Read the model definition and answer for the solid it produces. Units are mm, in the model's axes. A direction names the side the tool comes from. Give positions to 0.01 mm unless a question says otherwise; leave off trailing zeros. Write each loop counter-clockwise with the first axis right and the second up, starting at its lowest first coordinate (ties: lowest second). Pieces come first, ordered by that corner, then holes. Notation, with made-up numbers: (-22.5, -35) -> (26.5, -35) arc R11 cw to (26.5, -21) -> close; hole circle Ø4 at (60.25, 66). An arc over 180 degrees is marked (long way). Use a Markdown table: item, result.
from build123d import *

# Parameters (mm, degrees)
SKETCH_1_R          = 1.7
EXTRUDE_1_DEPTH     = 10
SKETCH_2_R          = 1.7
EXTRUDE_2_DEPTH     = 2.5
FILLET_1_R          = 9.5
FILLET_2_R          = 9.5
FILLET_3_R          = 9.5
SKETCH_3_R          = 5
SKETCH_3_R_2        = 3
EXTRUDE_3_DEPTH     = 3
CUT_EXTRUDE_1_DEPTH = 0.4
CUT_EXTRUDE_2_DEPTH = 3
SKETCH_6_W          = 8
SKETCH_6_H          = 9.5
SKETCH_6_W_2        = 2.5
SKETCH_6_H_2        = 30
EXTRUDE_4_DEPTH     = 5
EXTRUDE_5_DEPTH     = 2
EXTRUDE_1_2_DEPTH   = 2
EXTRUDE_3_2_DEPTH   = 3
FILLET_4_R          = 1


with BuildPart() as part:
    # Эскиз1 → Extrude 1 (new body)
    with BuildSketch(Plane(origin=(0, 0, 0), x_dir=(1, 0, 0), z_dir=(0, 1, 0))):
        with BuildLine():
            ThreePointArc((-44.999265675, -44.551130115), (-44.120586019, -46.672450458), (-41.999265675, -47.551130115))
            Line((-41.999265675, -47.551130115), (40.500734325, -47.551130115))
            ThreePointArc((40.500734325, -47.551130115), (42.622054669, -46.672450458), (43.500734325, -44.551130115))
            Line((43.500734325, -44.551130115), (43.500734325, 45.448869885))
            ThreePointArc((43.500734325, 45.448869885), (42.622054669, 47.570190229), (40.500734325, 48.448869885))
            Line((40.500734325, 48.448869885), (-41.999265675, 48.448869885))
            ThreePointArc((-41.999265675, 48.448869885), (-44.120586019, 47.570190229), (-44.999265675, 45.448869885))
            Line((-44.999265675, 45.448869885), (-44.999265675, -44.551130115))
        make_face()
        with Locations((-40.599265675, -43.151130115)):
            Circle(SKETCH_1_R, mode=Mode.SUBTRACT)
        with Locations((-0.749265675, -43.151130115)):
            Circle(SKETCH_1_R, mode=Mode.SUBTRACT)
        with Locations((39.100734325, -43.151130115)):
            Circle(SKETCH_1_R, mode=Mode.SUBTRACT)
        with Locations((-40.599265675, 0.448869885)):
            Circle(SKETCH_1_R, mode=Mode.SUBTRACT)
        with Locations((-40.599265675, 44.048869885)):
            Circle(SKETCH_1_R, mode=Mode.SUBTRACT)
        with Locations((-0.749265675, 44.048869885)):
            Circle(SKETCH_1_R, mode=Mode.SUBTRACT)
        Polygon((-17.403857393, -29.173018851), (-17.403857393, -31.551130115), (-17.403857393, -39.173018851), (-36.903857393, -39.173018851), (-36.903857393, 41.326981149), (-17.403857393, 41.326981149), (-17.403857393, 40.448869885), (-17.403857393, 31.326981149), (-15.999265675, 31.326981149), (-15.999265675, 40.448869885), (38.000734325, 40.448869885), (38.000734325, 10.448869885), (35.500734325, 10.448869885), (35.500734325, -29.051130115), (35.500734325, -30.051130115), (35.500734325, -39.551130115), (27.500734325, -39.551130115), (27.500734325, -30.051130115), (21.000734325, -30.051130115), (21.000734325, -31.551130115), (-15.999265675, -31.551130115), (-15.999265675, -29.173018851), align=None, mode=Mode.SUBTRACT)
        with Locations((39.100734325, 0.448869885)):
            Circle(SKETCH_1_R, mode=Mode.SUBTRACT)
        with Locations((39.100734325, 44.048869885)):
            Circle(SKETCH_1_R, mode=Mode.SUBTRACT)
    extrude(amount=EXTRUDE_1_DEPTH)

    # Эскиз2 → Бобышка-Вытянуть2 (add)
    with BuildSketch(Plane(origin=(0, 10, 0), x_dir=(1, 0, 0), z_dir=(0, 1, 0))):
        with BuildLine():
            Line((43.500734325, 45.448869885), (43.500734325, -44.551130115))
            ThreePointArc((43.500734325, -44.551130115), (42.622054669, -46.672450458), (40.500734325, -47.551130115))
            Line((40.500734325, -47.551130115), (-41.999265675, -47.551130115))
            ThreePointArc((-41.999265675, -47.551130115), (-44.120586019, -46.672450458), (-44.999265675, -44.551130115))
            Line((-44.999265675, -44.551130115), (-44.999265675, 45.448869885))
            ThreePointArc((-44.999265675, 45.448869885), (-44.120586019, 47.570190229), (-41.999265675, 48.448869885))
            Line((-41.999265675, 48.448869885), (40.500734325, 48.448869885))
            ThreePointArc((40.500734325, 48.448869885), (42.622054669, 47.570190229), (43.500734325, 45.448869885))
        make_face()
        with Locations((39.100734325, 0.448869885)):
            Circle(SKETCH_2_R, mode=Mode.SUBTRACT)
        with Locations((39.100734325, -43.151130115)):
            Circle(SKETCH_2_R, mode=Mode.SUBTRACT)
        with Locations((-0.749265675, -43.151130115)):
            Circle(SKETCH_2_R, mode=Mode.SUBTRACT)
        with Locations((-40.599265675, -43.151130115)):
            Circle(SKETCH_2_R, mode=Mode.SUBTRACT)
        with Locations((-40.599265675, 0.448869885)):
            Circle(SKETCH_2_R, mode=Mode.SUBTRACT)
        with Locations((39.100734325, 44.048869885)):
            Circle(SKETCH_2_R, mode=Mode.SUBTRACT)
        with Locations((-0.749265675, 44.048869885)):
            Circle(SKETCH_2_R, mode=Mode.SUBTRACT)
        with Locations((-40.599265675, 44.048869885)):
            Circle(SKETCH_2_R, mode=Mode.SUBTRACT)
    extrude(amount=EXTRUDE_2_DEPTH)

    # Скругление1
    fillet_1_edges = [part.edges().sort_by_distance(p)[0] for p in [
        (-36.903857393, 10, -1.076981149),
    ]]
    fillet(fillet_1_edges, radius=FILLET_1_R)

    # Скругление2
    fillet_2_edges = [part.edges().sort_by_distance(p)[0] for p in [
        (-17.403857393, 10, 34.173018851),
    ]]
    fillet(fillet_2_edges, radius=FILLET_2_R)

    # Скругление3
    fillet_3_edges = [part.edges().sort_by_distance(p)[0] for p in [
        (-17.403857393, 10, -36.326981149),
    ]]
    fillet(fillet_3_edges, radius=FILLET_3_R)

    # Эскиз3 → Extrude 3 (add)
    with BuildSketch(Plane.XZ.offset(-10)):
        with Locations((9.100734325, -2.448869885)):
            Circle(SKETCH_3_R)
        with Locations((9.100734325, -2.448869885)):
            Circle(SKETCH_3_R_2, mode=Mode.SUBTRACT)
    extrude(amount=EXTRUDE_3_DEPTH)

    # Эскиз4 → Вырез-Вытянуть1 (cut)
    with BuildSketch(Plane(origin=(0, 12.5, 0), x_dir=(1, 0, 0), z_dir=(0, 1, 0))):
        with BuildLine():
            Line((6.592743591, 7.281943928), (6.592743591, 4.666551979))
            ThreePointArc((6.592743591, 4.666551979), (3.388096655, 0), (6.592743591, -4.666551979))
            Line((6.592743591, -4.666551979), (6.592743591, -7.281943928))
            ThreePointArc((6.592743591, -7.281943928), (0.888096655, 0), (6.592743591, 7.281943928))
        make_face()
        with BuildLine():
            Line((10.18344972, 7.281943928), (10.18344972, 4.666551979))
            ThreePointArc((10.18344972, 4.666551979), (13.388096655, 0), (10.18344972, -4.666551979))
            Line((10.18344972, -4.666551979), (10.18344972, -7.281943928))
            ThreePointArc((10.18344972, -7.281943928), (15.888096655, 0), (10.18344972, 7.281943928))
        make_face()
    extrude(amount=-CUT_EXTRUDE_1_DEPTH, mode=Mode.SUBTRACT)

    # Эскиз5 → Вырез-Вытянуть2 (cut)
    with BuildSketch(Plane(origin=(0, 12.5, 0), x_dir=(1, 0, 0), z_dir=(0, 1, 0))):
        Polygon((-40.599265675, 40.700238324), (-37.699265675, 42.374554105), (-37.699265675, 45.723185666), (-40.599265675, 47.397501447), (-43.499265675, 45.723185666), (-43.499265675, 42.374554105), align=None)
        Polygon((-0.749265675, 40.700238324), (2.150734325, 42.374554105), (2.150734325, 45.723185666), (-0.749265675, 47.397501447), (-3.649265675, 45.723185666), (-3.649265675, 42.374554105), align=None)
        Polygon((-40.599265675, 3.797501447), (-43.499265675, 2.123185666), (-43.499265675, -1.225445895), (-40.599265675, -2.899761676), (-37.699265675, -1.225445895), (-37.699265675, 2.123185666), align=None)
        Polygon((36.200734325, 2.123185666), (39.100734325, 3.797501447), (42.000734325, 2.123185666), (42.000734325, -1.225445895), (39.100734325, -2.899761676), (36.200734325, -1.225445895), align=None)
        Polygon((42.000734325, 42.374554105), (39.100734325, 40.700238324), (36.200734325, 42.374554105), (36.200734325, 45.723185666), (39.100734325, 47.397501447), (42.000734325, 45.723185666), align=None)
        Polygon((39.100734325, -39.802498553), (36.200734325, -41.476814334), (36.200734325, -44.825445895), (39.100734325, -46.499761676), (42.000734325, -44.825445895), (42.000734325, -41.476814334), align=None)
        Polygon((-3.649265675, -41.476814334), (-0.749265675, -39.802498553), (2.150734325, -41.476814334), (2.150734325, -44.825445895), (-0.749265675, -46.499761676), (-3.649265675, -44.825445895), align=None)
        Polygon((-43.499265675, -41.476814334), (-40.599265675, -39.802498553), (-37.699265675, -41.476814334), (-37.699265675, -44.825445895), (-40.599265675, -46.499761676), (-43.499265675, -44.825445895), align=None)
    extrude(amount=-CUT_EXTRUDE_2_DEPTH, mode=Mode.SUBTRACT)

    # Эскиз6 → Бобышка-Вытянуть4 (add)
    with BuildSketch(Plane.XZ.offset(-10)):
        with Locations((31.500734325, 34.801130115)):
            Rectangle(SKETCH_6_W, SKETCH_6_H)
        with Locations((36.750734325, -25.448869885)):
            Rectangle(SKETCH_6_W_2, SKETCH_6_H_2)
    extrude(amount=EXTRUDE_4_DEPTH)

    # Эскиз8 → Бобышка-Вытянуть5 (add)
    with BuildSketch(Plane.XZ.offset(-10)):
        with BuildLine():
            Line((35.500734325, -5.248869885), (35.500734325, 4.351130115))
            ThreePointArc((35.500734325, 4.351130115), (33.100734325, -0.448869885), (35.500734325, -5.248869885))
        make_face()
        with BuildLine():
            Line((-5.549265675, -40.448869885), (4.050734325, -40.448869885))
            ThreePointArc((4.050734325, -40.448869885), (-0.749265675, -38.048869885), (-5.549265675, -40.448869885))
        make_face()
    extrude(amount=EXTRUDE_5_DEPTH)

    # Эскиз9 → Extrude 1 2 (add)
    with BuildSketch(Plane.XZ):
        with BuildLine():
            Line((-44.999265675, 44.551130115), (-44.999265675, -45.448869885))
            ThreePointArc((-44.999265675, -45.448869885), (-44.120586019, -47.570190229), (-41.999265675, -48.448869885))
            Line((-41.999265675, -48.448869885), (40.500734325, -48.448869885))
            ThreePointArc((40.500734325, -48.448869885), (42.622054669, -47.570190229), (43.500734325, -45.448869885))
            Line((43.500734325, -45.448869885), (43.500734325, 44.551130115))
            ThreePointArc((43.500734325, 44.551130115), (42.622054669, 46.672450458), (40.500734325, 47.551130115))
            Line((40.500734325, 47.551130115), (-41.999265675, 47.551130115))
            ThreePointArc((-41.999265675, 47.551130115), (-44.120586019, 46.672450458), (-44.999265675, 44.551130115))
        make_face()
        with BuildLine():
            Line((-43.699265675, 44.551130115), (-43.699265675, -45.448869885))
            ThreePointArc((-43.699265675, -45.448869885), (-43.201347203, -46.650951413), (-41.999265675, -47.148869885))
            Line((-41.999265675, -47.148869885), (40.500734325, -47.148869885))
            ThreePointArc((40.500734325, -47.148869885), (41.702815853, -46.650951413), (42.200734325, -45.448869885))
            Line((42.200734325, -45.448869885), (42.200734325, 44.551130115))
            ThreePointArc((42.200734325, 44.551130115), (41.702815853, 45.753211643), (40.500734325, 46.251130115))
            Line((40.500734325, 46.251130115), (-41.999265675, 46.251130115))
            ThreePointArc((-41.999265675, 46.251130115), (-43.201347203, 45.753211643), (-43.699265675, 44.551130115))
        make_face(mode=Mode.SUBTRACT)
    extrude(amount=EXTRUDE_1_2_DEPTH)

    # Эскиз11 → Extrude 3 2 (add)
    with BuildSketch(Plane.XZ.offset(2)):
        with BuildLine():
            Line((-41.999265675, -49.648869885), (40.500734325, -49.648869885))
            ThreePointArc((40.500734325, -49.648869885), (43.470582806, -48.418718366), (44.700734325, -45.448869885))
            Line((44.700734325, -45.448869885), (44.700734325, 44.551130115))
            ThreePointArc((44.700734325, 44.551130115), (43.470582806, 47.520978596), (40.500734325, 48.751130115))
            Line((40.500734325, 48.751130115), (-41.999265675, 48.751130115))
            ThreePointArc((-41.999265675, 48.751130115), (-44.969114156, 47.520978596), (-46.199265675, 44.551130115))
            Line((-46.199265675, 44.551130115), (-46.199265675, -45.448869885))
            ThreePointArc((-46.199265675, -45.448869885), (-44.969114156, -48.418718366), (-41.999265675, -49.648869885))
        make_face()
        with BuildLine():
            Line((-41.999265675, -47.148869885), (40.500734325, -47.148869885))
            ThreePointArc((40.500734325, -47.148869885), (41.702815853, -46.650951413), (42.200734325, -45.448869885))
            Line((42.200734325, -45.448869885), (42.200734325, 44.551130115))
            ThreePointArc((42.200734325, 44.551130115), (41.702815853, 45.753211643), (40.500734325, 46.251130115))
            Line((40.500734325, 46.251130115), (-41.999265675, 46.251130115))
            ThreePointArc((-41.999265675, 46.251130115), (-43.201347203, 45.753211643), (-43.699265675, 44.551130115))
            Line((-43.699265675, 44.551130115), (-43.699265675, -45.448869885))
            ThreePointArc((-43.699265675, -45.448869885), (-43.201347203, -46.650951413), (-41.999265675, -47.148869885))
        make_face(mode=Mode.SUBTRACT)
    extrude(amount=-EXTRUDE_3_2_DEPTH)

    # Скругление4
    fillet_4_edges = [part.edges().sort_by_distance(p)[0] for p in [
        (42.622054669, 1, -47.570190229),
        (42.622054669, 1, 46.672450458),
        (-0.749265675, 1, 47.551130115),
        (-44.120586019, 1, 46.672450458),
        (-44.999265675, 1, -0.448869885),
        (-44.120586019, 1, -47.570190229),
        (-0.749265675, 1, -48.448869885),
        (43.500734325, 1, -0.448869885),
    ]]
    fillet(fillet_4_edges, radius=FILLET_4_R)


solid = part.part
Item 1: A cutting plane is placed at D-D (x = -23). Give the vertices of the cut face in (y, z), then the cut area to 3 significant figures.
Return value:
| item | result |
|---|---|
| outline | (-2, -49.65) -> (1, -49.65) -> (1, -49.45) arc R1 cw to (2, -48.45) -> (12.5, -48.45) -> (12.5, 47.55) -> (2, 47.55) arc R1 cw to (1, 48.55) -> (1, 48.75) -> (-2, 48.75) -> (-2, 46.25) -> (0, 46.25) -> (0, 39.17) -> (9.16, 39.17) -> (9.16, 29.17) -> (10, 29.17) -> (10, -31.33) -> (9.16, -31.33) -> (9.16, -41.33) -> (0, -41.33) -> (0, -47.15) -> (-2, -47.15) -> close |
| area | 425 mm^2 |
Item 2: A cutting plane is placed at B-B (x = -8.5). Give the vertices of the cut face in (y, z), then the cut area to 3 significant figures.
Return value:
| item | result |
|---|---|
| outline | (-2, -49.65) -> (1, -49.65) -> (1, -49.45) arc R1 cw to (2, -48.45) -> (12.5, -48.45) -> (12.5, 47.55) -> (2, 47.55) arc R1 cw to (1, 48.55) -> (1, 48.75) -> (-2, 48.75) -> (-2, 46.25) -> (0, 46.25) -> (0, 31.55) -> (10, 31.55) -> (10, -40.45) -> (0, -40.45) -> (0, -47.15) -> (-2, -47.15) -> close |
| area | 493 mm^2 |
Item 3: Each of these flat-tipped pins is pushed along its axis until it touches: P1, Ø2, axis at x = 5.5, y = 5, coming from the -Z side; P2, Ø0.7, axis at y = 7.5, z = 30.5, coming from the +X side; P3, Ø1, axis at y = 2, z = 34.5, coming from the +X side; P4, Ø6.5, axis at x = -41, z = -0.5, coming from the +Y side. Where does it stop, or does it pass through?
Return value:
| item | result |
|---|---|
| P1 | z = -48.45 |
| P2 | x = 43.5 |
| P3 | x = 43.63 |
| P4 | y = 12.5 |
Item 4: A cutting plane is placed at A-A (z = -12). Give the vertices of the cut face in (x, y).
Return value:
| item | result |
|---|---|
| outline | (-46.2, -2) -> (-43.7, -2) -> (-43.7, 0) -> (-36.9, 0) -> (-36.9, 0.5) arc R9.5 cw to (-27.4, 10) -> (35.5, 10) -> (35.5, 5) -> (38, 5) -> (38, 0) -> (42.2, 0) -> (42.2, -2) -> (44.7, -2) -> (44.7, 1) -> (44.5, 1) arc R1 cw to (43.5, 2) -> (43.5, 12.5) -> (-45, 12.5) -> (-45, 2) arc R1 cw to (-46, 1) -> (-46.2, 1) -> close |
Item 5: A cutting plane is placed at C-C (z = 20). Give the vertices of the cut face in (x, y), then the cut area to 3 significant figures.
Return value:
| item | result |
|---|---|
| outline | (-46.2, -2) -> (-43.7, -2) -> (-43.7, 0) -> (-36.9, 0) -> (-36.9, 0.5) arc R9.5 cw to (-27.4, 10) -> (35.5, 10) -> (35.5, 0) -> (42.2, 0) -> (42.2, -2) -> (44.7, -2) -> (44.7, 1) -> (44.5, 1) arc R1 cw to (43.5, 2) -> (43.5, 12.5) -> (-45, 12.5) -> (-45, 2) arc R1 cw to (-46, 1) -> (-46.2, 1) -> close |
| area | 414 mm^2 |
Item 6: A tool of negligible diameter and unlimited length cuts with its end or side. For faces 3 (the face through (32, 2, 39.551)), 4 (the face through (-44.097, 7.324, 46.696)), 5 (the face through (0.72, 11.02, 45.65)), from which of +Z, -Z, +X, -X, +Y, -Y can it reach the whole face along a straight path? Write none if from no direction.
Return value:
| item | result |
|---|---|
| face 3 | -Y |
| face 4 | +Z, -X, +Y |
| face 5 | +Y |
Item 7: Straight lines are drawn through the part: line 1 along X through (y, z) = (0.75, 36); line 2 along Z through (x, y) = (-21.5, 7); line 3 along Z through (x, y) = (-17, 9.25). For each, find the intervals that lie inside material, in ascending order. Write a range as [from, to].
Return value:
| item | result |
|---|---|
| line 1 | [-46.2, -36.9], [-17.41, 27.5], [35.5, 44.7] |
| line 2 | [-48.45, -41.33], [39.17, 47.55] |
| line 3 | [-48.45, -31.33], [29.17, 47.55] |
Item 8: For a pull along Z with two mould halves and no side action, classify faces 1 (the face through (0.5, 9.5, -42.6)), 2 (the face through (43.5, -0.52, 47.49)) as +Z half, -Z half, draft (parallel to the pull), parting line (faces both ways), or undercut.
Return value:
| item | result |
|---|---|
| face 1 | undercut |
| face 2 | +Z half |
